from build123d import *

# Parameters (mm, degrees)
SKETCH1_W               = 75
SKETCH1_H               = 75
SKETCH1_R               = 2.75
SKETCH1_R_2             = 5
BOSS_EXTRUDE1_DEPTH     = 3.175
CUT_EXTRUDE1_DEPTH      = 320.126840966
CUT_EXTRUDE1_DEPTH_BACK = 320.126840966
FILLET1_R               = 10


with BuildPart() as part:
    # Sketch1 → Boss-Extrude1 (new body)
    with BuildSketch(Plane.XY.offset(151.125)):
        with Locations((0, 279.4)):
            Rectangle(SKETCH1_W, SKETCH1_H)
        with Locations((-27.5, 251.9)):
            Circle(SKETCH1_R, mode=Mode.SUBTRACT)
        with Locations((27.5, 251.9)):
            Circle(SKETCH1_R, mode=Mode.SUBTRACT)
        with Locations((27.5, 306.9)):
            Circle(SKETCH1_R, mode=Mode.SUBTRACT)
        with Locations((-27.5, 306.9)):
            Circle(SKETCH1_R, mode=Mode.SUBTRACT)
        with Locations((0, 279.4)):
            Circle(SKETCH1_R_2, mode=Mode.SUBTRACT)
    extrude(amount=BOSS_EXTRUDE1_DEPTH)

    # Sketch2 → Cut-Extrude1 (cut, two sides: drawn at the far end of the back side and taken through both)
    with BuildSketch(Plane.XY.offset(154.3).offset(-CUT_EXTRUDE1_DEPTH_BACK)):
        with BuildLine():
            Line((5.656854249, 287.178174593), (9.545941546, 291.06726189))
            ThreePointArc((9.545941546, 291.06726189), (11.66726189, 291.06726189), (11.66726189, 288.945941546))
            Line((11.66726189, 288.945941546), (7.778174593, 285.056854249))
            ThreePointArc((7.778174593, 285.056854249), (5.656854249, 285.056854249), (5.656854249, 287.178174593))
        make_face()
        with BuildLine():
            Line((7.778174593, 273.743145751), (11.66726189, 269.854058454))
            ThreePointArc((11.66726189, 269.854058454), (11.66726189, 267.73273811), (9.545941546, 267.73273811))
            Line((9.545941546, 267.73273811), (5.656854249, 271.621825407))
            ThreePointArc((5.656854249, 271.621825407), (5.656854249, 273.743145751), (7.778174593, 273.743145751))
        make_face()
        with BuildLine():
            Line((-5.656854249, 271.621825407), (-9.545941546, 267.73273811))
            ThreePointArc((-9.545941546, 267.73273811), (-11.66726189, 267.73273811), (-11.66726189, 269.854058454))
            Line((-11.66726189, 269.854058454), (-7.778174593, 273.743145751))
            ThreePointArc((-7.778174593, 273.743145751), (-5.656854249, 273.743145751), (-5.656854249, 271.621825407))
        make_face()
        with BuildLine():
            Line((-7.778174593, 285.056854249), (-11.66726189, 288.945941546))
            ThreePointArc((-11.66726189, 288.945941546), (-11.66726189, 291.06726189), (-9.545941546, 291.06726189))
            Line((-9.545941546, 291.06726189), (-5.656854249, 287.178174593))
            ThreePointArc((-5.656854249, 287.178174593), (-5.656854249, 285.056854249), (-7.778174593, 285.056854249))
        make_face()
    extrude(amount=CUT_EXTRUDE1_DEPTH + CUT_EXTRUDE1_DEPTH_BACK, mode=Mode.SUBTRACT)

    # Fillet1
    fillet1_edges = [part.edges().sort_by_distance(p)[0] for p in [
        (37.5, 241.9, 152.7125),
        (-37.5, 241.9, 152.7125),
        (-37.5, 316.9, 152.7125),
        (37.5, 316.9, 152.7125),
    ]]
    fillet(fillet1_edges, radius=FILLET1_R)


solid = part.part
Part model, mm, in its own coordinate system. A direction names the side the tool comes from. Coordinates: 2 decimals unless noted, no trailing zeros. Loops run counter-clockwise (first coordinate to the right, second up) from the corner with the lowest first, then second, coordinate; pieces in that order, holes last. Notation, with made-up numbers: (70, 8) - (118, 8) arc R23 cw to (118, 26) - close; hole circle Ø6 at (76, 56). An arc over 180 degrees is marked (long way). Write each question's results on one line, items separated by ' | '. Start each with the question number.
Q1. Drop a flat-ended pin along its axis: pin 1 Ø3.5 at (x, y) = (-27.5, 306.9) entering from -Z. Give the stop position or say it passes through.
Q2. Which spindle directions (+Z, -Z, +X, -X, +Y, -Y) get a long thin tool onto all of the face, cutting with end or side? Do faces 1 (the flat face through (0, 241.9, 153)), 2 (the flat face through (-9.695, 286.974, 152.69)). Say none if no direction does.
Q3. Two-plate mould, pull along Y, no slides. Class faces 3 (the flat face through (-1, 288, 154.3)), 4 (the cylindrical face through (-34.65, 313.89, 152.73)), 5 (the flat face through (-7.63, 289.15, 152.69)), 6 (the flat face through (9.695, 271.826, 152.69)): +Y half, -Y half, draft (parallel to the pull), parting line (faces both ways), or undercut.
Q4. Slice it at D-D on y = 312. Give the cut face in (x, z) (3 decimals), and give its area (3 significant figures).
Q5. Slice it at B-B on z = 151.8. Give the number of separate pieces and of enclosed holes in the cut face, and give its area (3 significant figures).
Q6. Probe line 1 along X through (y, z) = (306.9, 152.9); line 2 along Y through (x, z) = (-27.5, 153); line 3 along X through (y, z) = (279.4, 153.5). List the from-to ranges inside material, lowest first.
Q7. Slice it at C-C on x = 26.5. Give the cut face in (y, z) (3 decimals).
Q8. Slice it at A-A on y = 279.4. Give the cut face in (x, z) (3 decimals), and give its area (3 significant figures).
Answer:
1) pin 1: passes through
2) face 1: +Z, -Z, +X, -X, -Y | face 2: +Z, -Z
3) face 3: draft | face 4: +Y half | face 5: undercut | face 6: undercut
4) outline: (-36.102, 151.125) - (36.102, 151.125) - (36.102, 154.3) - (-36.102, 154.3) - close | area: 229 mm2
5) separate pieces: 1 | enclosed holes: 9 | area: 5,270 mm2
6) line 1: x = -37.5 to -30.25, -24.75 to 24.75, 30.25 to 37.5 | line 2: y = 241.9 to 249.15, 254.65 to 304.15, 309.65 to 316.9 | line 3: x = -37.5 to -5, 5 to 37.5
7) outline: (241.9, 151.125) - (249.338, 151.125) - (249.338, 154.3) - (241.9, 154.3) - close; (254.462, 151.125) - (304.338, 151.125) - (304.338, 154.3) - (254.462, 154.3) - close; (309.462, 151.125) - (316.9, 151.125) - (316.9, 154.3) - (309.462, 154.3) - close
8) outline: (-37.5, 151.125) - (-5, 151.125) - (-5, 154.3) - (-37.5, 154.3) - close; (5, 151.125) - (37.5, 151.125) - (37.5, 154.3) - (5, 154.3) - close | area: 206 mm2
